```python
from build123d import *

# Parameters (mm, degrees)
BOSS_EXTRUDE1_DEPTH = 4.8


with BuildPart() as part:
    # Sketch1 → Boss-Extrude1 (new body)
    with BuildSketch(Plane(origin=(0, 0, 0), x_dir=(1, 0, 0), z_dir=(0, 1, 0))):
        with BuildLine():
            Line((18, 3.5), (18, 2.5))
            ThreePointArc((18, 2.5), (17.581582801, 1.460683569), (16.559761807, 1.001190964))
            Line((16.559761807, 1.001190964), (3.980079398, 0.499603012))
            ThreePointArc((3.980079398, 0.499603012), (3.5, 0), (3.980079398, -0.499603012))
            Line((3.980079398, -0.499603012), (16.559761807, -1.001190964))
            ThreePointArc((16.559761807, -1.001190964), (17.581582801, -1.460683569), (18, -2.5))
            Line((18, -2.5), (18, -3.5))
            ThreePointArc((18, -3.5), (17.414213562, -4.914213562), (16, -5.5))
            Line((16, -5.5), (-16, -5.5))
            ThreePointArc((-16, -5.5), (-17.414213562, -4.914213562), (-18, -3.5))
            Line((-18, -3.5), (-18, -2.5))
            ThreePointArc((-18, -2.5), (-17.581582801, -1.460683569), (-16.559761807, -1.001190964))
            Line((-16.559761807, -1.001190964), (-3.980079398, -0.499603012))
            ThreePointArc((-3.980079398, -0.499603012), (-3.5, 0), (-3.980079398, 0.499603012))
            Line((-3.980079398, 0.499603012), (-16.559761807, 1.001190964))
            ThreePointArc((-16.559761807, 1.001190964), (-17.581582801, 1.460683569), (-18, 2.5))
            Line((-18, 2.5), (-18, 3.5))
            ThreePointArc((-18, 3.5), (-17.414213562, 4.914213562), (-16, 5.5))
            Line((-16, 5.5), (16, 5.5))
            ThreePointArc((16, 5.5), (17.414213562, 4.914213562), (18, 3.5))
        make_face()
        with BuildLine():
            Line((16.5, 3.5), (-16.5, 3.5))
            Line((-16.5, 3.5), (-16.5, 2.5))
            Line((-16.5, 2.5), (-3.92031759, 1.998412048))
            ThreePointArc((-3.92031759, 1.998412048), (-2, 0), (-3.92031759, -1.998412048))
            Line((-3.92031759, -1.998412048), (-16.5, -2.5))
            Line((-16.5, -2.5), (-16.5, -3.5))
            Line((-16.5, -3.5), (16.5, -3.5))
            Line((16.5, -3.5), (16.5, -2.5))
            Line((16.5, -2.5), (3.92031759, -1.998412048))
            ThreePointArc((3.92031759, -1.998412048), (2, 0), (3.92031759, 1.998412048))
            Line((3.92031759, 1.998412048), (16.5, 2.5))
            Line((16.5, 2.5), (16.5, 3.5))
        make_face(mode=Mode.SUBTRACT)
    extrude(amount=BOSS_EXTRUDE1_DEPTH)


solid = part.part
```
Design review of the part built by this model. Coordinates are the model's own, in mm. A direction names the side the tool comes from. Give positions to 0.01 mm unless a question says otherwise; leave off trailing zeros. Write each loop counter-clockwise with the first axis right and the second up, starting at its lowest first coordinate (ties: lowest second). Pieces come first, ordered by that corner, then holes. Notation, with made-up numbers: (54.25, 61.5) -> (106.25, 61.5) arc R23 ccw to (106.25, 77.5) -> close; hole circle Ø9 at (87.25, 58.5). An arc over 180 degrees is marked (long way). Answer in a Markdown table with one row per item.
(1) Mouldability with a two-part tool opening along Z and no side actions: class faces 4 (the flat face through (0, 2, -5.5)), 5 (the flat face through (16.5, 2, 3)), 6 (the flat face through (18, 2, 3)), 7 (the cylindrical face through (-17.59, 2.37, 1.47)) as +Z half, -Z half, draft (parallel to the pull), parting line (faces both ways), or undercut.
Results:
| item | result |
|---|---|
| face 4 | -Z half |
| face 5 | undercut |
| face 6 | draft |
| face 7 | undercut |
(2) Consider section C-C (x = 11). State the section outline as (y, z) points, then the cut area to 3 significant figures.
Results:
| item | result |
|---|---|
| outline | (0, -5.5) -> (4.8, -5.5) -> (4.8, -3.5) -> (0, -3.5) -> close; (0, -2.28) -> (4.8, -2.28) -> (4.8, -0.78) -> (0, -0.78) -> close; (0, 0.78) -> (4.8, 0.78) -> (4.8, 2.28) -> (0, 2.28) -> close; (0, 3.5) -> (4.8, 3.5) -> (4.8, 5.5) -> (0, 5.5) -> close |
| area | 33.6 mm2 |
(3) For faces 1 (the flat face through (-10.298, 2.366, -2.253)), 2 (the cylindrical face through (17.57, 2.37, 1.45)), 3 (the flat face through (-10.182, 2.366, -0.747)), list the 3-axis set-ups (+Z, -Z, +X, -X, +Y, -Y) from which the entire face can be reached by the end or side of a thin tool; tool diameter is ignored.
Results:
| item | result |
|---|---|
| face 1 | +Y, -Y |
| face 2 | +X, +Y, -Y |
| face 3 | -X, +Y, -Y |
(4) Consider section A-A (z = 3). State the section outline as (x, y) points.
Results:
| item | result |
|---|---|
| outline | (-18, 0) -> (-16.5, 0) -> (-16.5, 4.8) -> (-18, 4.8) -> close; (16.5, 0) -> (18, 0) -> (18, 4.8) -> (16.5, 4.8) -> close |
(5) To check wall thickness, follow probe 1 along Z at (x, y) = (-4, 4.3); probe 2 along X at (y, z) = (2.25, -3.25); probe 3 along Z at (x, y) = (-10, 2.45). State the ranges of each line that lie inside material, in increasing order.
Results:
| item | result |
|---|---|
| probe 1 | -5.5 to -3.5, -2 to -0.5, 0.5 to 2, 3.5 to 5.5 |
| probe 2 | -18 to -16.5, 16.5 to 18 |
| probe 3 | -5.5 to -3.5, -2.24 to -0.74, 0.74 to 2.24, 3.5 to 5.5 |
(6) Clearance check with flat-ended pins moving along their axes: pin 1 (1.5 mm diameter, centred on y = 3, z = 4.5, fed in from +X); pin 2 (1.5 mm diameter, centred on x = 0, z = 0.5, fed in from -Y). State where each tip first meets the part, or that it passes through.
Results:
| item | result |
|---|---|
| pin 1 | x = 17.98 |
| pin 2 | through |
